Autodesk Inventor part; units mm, degrees
ref_plane "YZ Plane" through (0, 0, 0) normal (1, 0, 0) x (0, 1, 0)
ref_plane "XZ Plane" through (0, 0, 0) normal (0, 1, 0) x (-1, 0, 0)
ref_plane "XY Plane" through (0, 0, 0) normal (0, 0, 1) x (1, 0, 0)
sketch "Sketch1" plane through (0, 0, 0) normal (0, 1, 0) x (-1, 0, 0)
  line L0 (0, -27.8975) -> (20, -27.8975)
  line L1 (20, -27.8975) -> (20, -53.2975)
  line L2 (20, -53.2975) -> (0, -53.2975)
  line L3 (0, -53.2975) -> (0, -27.8975)
  point P0 (0, 0)
  dimension "d0" = 20
  dimension "d1" = 25.4
extrude "Extrusion1" add sketch "Sketch1" along normal blind 2.54
sketch "Sketch2" plane through (0, 0, -27.8975) normal (1, 0, 0) x (0, 0, -1)
  line L0 (0, 0) -> (25.4, 0)
  line L1 (0, 2.54) -> (25.4, 2.54)
  line L2 (25.4, 2.54) -> (25.4, 0)
  line L3 (25.4, 0) -> (0, 0)
  line L4 (0, 0) -> (0, 2.54)
  point P0 (-27.8975, 0)
extrude "Extrusion2" add sketch "Sketch2" along normal blind 5.08
sketch "Sketch4" plane through (-20, 0, -27.8975) normal (0, 0, 1) x (1, 0, 0)
  line L0 (25.08, 2.54) -> (25.08, 0) construction
  line L1 (25.08, 2.54) -> (20, 2.54) construction
  line L2 (0, 0) -> (25.08, 0)
  line L3 (25.08, 0) -> (20, 0)
  line L4 (0, 2.54) -> (25.08, 2.54)
  line L5 (25.08, 2.54) -> (25.08, 10.16)
  line L6 (25.08, 0) -> (25.08, -7.62)
  line L7 (20, 2.54) -> (25.08, 10.16)
  line L8 (20, 0) -> (25.08, -7.62)
  line L9 (25.08, 10.16) -> (40.32, 10.16)
  line L10 (40.32, 10.16) -> (40.32, 7.628)
  line L11 (25.08, 8.898) -> (25.08, 10.16)
  line L12 (25.08, -7.62) -> (40.32, -7.62)
  line L13 (40.32, -7.62) -> (40.32, -7.6153)
  line L14 (25.08, -7.6153) -> (25.08, -7.62)
  line L15 (40.32, 10.16) -> (42.8586, 10.16)
  line L16 (42.8586, 10.16) -> (42.8586, -7.62)
  line L17 (42.8586, -7.62) -> (40.32, -7.62)
  line L18 (40.32, -7.62) -> (40.32, 10.16)
  line L19 (40.32, -7.6177) -> (25.08, -7.6177)
  line L20 (40.32, -7.6177) -> (25.08, -7.6177)
  line L21 (25.08, -7.6177) -> (25.08, -6.3417)
  line L22 (25.08, -6.3417) -> (40.32, -6.3417)
  line L23 (40.32, -6.3417) -> (40.32, -7.6177)
  line L24 (40.32, 10.16) -> (25.08, 10.16)
  line L25 (25.08, 10.16) -> (25.08, 8.898)
  line L26 (25.08, 8.898) -> (40.32, 8.898)
  line L27 (40.32, 8.898) -> (40.32, 10.16)
  line L28 (32.7, 8.898) -> (30.1596, 8.898)
  line L29 (30.1596, 8.898) -> (30.1596, -6.3417)
  line L30 (30.1596, -6.3417) -> (32.7, -6.3417)
  line L31 (32.7, -6.3417) -> (32.7, 8.898)
  dimension "d6" = 7.62
  dimension "d7" = 2.54
  dimension "d9" = 7.62
  dimension "d10" = 15.24
  dimension "d16" = 15.24
  dimension "d30" = 17.78
extrude "Extrusion3" add sketch "Sketch4" against normal blind 25.4 contours L2 L6 L8 | L6 L22 L18 L13 L19 | L13 L18 L10 L15 L16 L17 | L29 L26 L31 L22 | L26 L5 L9 L10 | L5 L4 L7
sketch "Sketch6" plane through (22.8586, -7.62, -27.8975) normal (1, 0, 0) x (0, 0, -1)
  line L0 (25.4, 10.16) -> (25.4, 17.78)
  line L1 (0, 7.62) -> (0, 0)
  line L2 (25.4, 17.78) -> (0, 17.78)
  line L3 (0, 17.78) -> (0, 0)
  line L4 (0, 0) -> (25.4, 0)
  line L5 (25.4, 0) -> (25.4, 17.78)
  line L6 (0, 17.78) -> (0, 10.16)
  line L7 (25.4, 0) -> (0, 17.78)
  line L8 (0, 0) -> (25.4, 17.78)
  circle A0 centre (12.7, 8.89) radius 1.905
  point P0 (-27.8975, 7.62)
  dimension "d17" = 3.81
extrude "Extrusion5" cut sketch "Sketch6" against normal blind 14.2875 contours A0 L7 L8 | L8 L7 A0 | A0 L8 L7 | L7 L8 A0
sketch "Sketch8" plane through (-20, 0, -27.8975) normal (0, 0, 1) x (1, 0, 0)
  line L0 (0, 0) -> (20, 0)
  line L1 (0, 2.54) -> (20, 2.54)
  line L2 (0, 0) -> (20, 0)
  line L3 (20, 0) -> (20, 2.54)
  line L4 (20, 2.54) -> (0, 2.54)
  line L5 (0, 2.54) -> (0, 0)
extrude "Extrusion7" add sketch "Sketch8" along normal blind 50.8
sketch "Sketch10" plane through (0, 2.54, 0) normal (0, 1, 0) x (1, 0, 0)
  circle A0 centre (-10.4728, -4.8164) radius 9.779
  circle A1 centre (-10.4728, -14.5954) radius 1.905
  circle A2 centre (-10.4728, 4.9626) radius 1.905
  point P0 (0, 0)
  dimension "d31" = 19.558
  dimension "d32" = 3.81
  dimension "d33" = 3.81
extrude "Extrusion9" cut sketch "Sketch10" against normal blind 50.8 contours A2 A0 | A0 A2 | A1 A0 | A0 A1
properties part number "VbearingBracket"
Could you check a few things on this model? Use its own coordinates, in mm. A direction names the side the tool comes from. Give positions to 0.01 mm unless a question says otherwise; leave off trailing zeros. Order: outer loops, then holes, each group sorted by start corner. A loop starts at its lowest first (then second) coordinate and runs counter-clockwise, first axis right, second up. Notation, with made-up numbers: (-38.5, 52.5) -> (-3.5, 52.5) arc R13 cw to (-3.5, 72.5) -> close; hole circle Ø7 at (6, 5). An arc over 180 degrees is marked (long way). Answer in a Markdown table with one row per item. Add a question column.
Item 1: I'm going to push flat-ended pins straight in: P1, Ø16, axis at x = -9, z = 5.5, coming from the +Y side; P2, Ø3, axis at x = 1, z = -29, coming from the +Y side; P3, Ø3.5, axis at x = -10.47, z = 14.6, coming from the -Y side; P4, Ø2, axis at x = 3, y = 1, coming from the +Z side. Where does each tip first touch, or does it pass through?
Item 2: Imagine slicing it at A-A (x = 16). List the corners of the cut face in (y, z) for me.
Item 3: Please list where these lines run through material, in increasing order: probe 1 along X at (y, z) = (-3, -37.5); probe 2 along Y at (x, z) = (19.5, -29); probe 3 along Y at (x, z) = (-3.5, -36.5).
Item 4: Imagine slicing it at B-B (y = -4.5). List the corners of the cut face in (x, z) for me, and give its area (3 significant figures).
Item 5: We'd pull the mould along Y, two halves only. Please class faces 4 (the flat face through (0, 1, -3)), 5 (the flat face through (8, -6.342, -40)), 6 (the flat face through (2.504, 6.297, -40.42)): pulls with the +Y half, pulls with the -Y half, needs draft (parallel to the pull), parting line crosses it, or undercut.
Item 6: Imagine slicing it at D-D (z = 2). List the corners of the cut face in (x, y) for me.
Item 7: For faces 1 (the flat face through (8, 8.898, -40)), 2 (the flat face through (13, -7.618, -40)), 3 (the cylindrical face through (11.448, 1.842, -42.415)), which set-ups out of +Z, -Z, +X, -X, +Y, -Y let a thin tool reach every point of the face, with its end or its side?
Item 8: Imagine slicing it at C-C (y = 1.27). List the corners of the cut face in (x, z) for me (1 decimal).
Result:
| question | item | result |
|---|---|---|
| 1 | P1 | y = 2.54 |
| 1 | P2 | y = 6.29 |
| 1 | P3 | through |
| 1 | P4 | z = -27.9 |
| 2 | outline | (-7.62, -53.3) -> (-6.34, -53.3) -> (-6.34, -27.9) -> (-7.62, -27.9) -> close; (8.9, -53.3) -> (10.16, -53.3) -> (10.16, -27.9) -> (8.9, -27.9) -> close |
| 3 | probe 1 | 2 to 5.08, 10.16 to 12.7, 20.32 to 22.86 |
| 3 | probe 2 | -7.62 to -6.34, 8.9 to 10.16 |
| 3 | probe 3 | 0 to 2.54 |
| 4 | outline | (3, -53.3) -> (5.08, -53.3) -> (5.08, -27.9) -> (3, -27.9) -> close; (10.16, -53.3) -> (12.7, -53.3) -> (12.7, -27.9) -> (10.16, -27.9) -> close; (20.32, -53.3) -> (22.86, -53.3) -> (22.86, -27.9) -> (20.32, -27.9) -> close |
| 4 | area | 182 mm2 |
| 5 | face 4 | needs draft |
| 5 | face 5 | undercut |
| 5 | face 6 | pulls with the +Y half |
| 6 | outline | (-20, 0) -> (0, 0) -> (0, 2.54) -> (-20, 2.54) -> close |
| 7 | face 1 | +Z, -Z |
| 7 | face 2 | +Z, -Z, +X, -X, -Y |
| 7 | face 3 | +X |
| 8 | outline | (-20, -53.3) -> (5.1, -53.3) -> (5.1, -27.9) -> (0, -27.9) -> (0, 22.9) -> (-20, 22.9) -> close; (10.2, -53.3) -> (12.7, -53.3) -> (12.7, -42.5) -> (10.2, -42.5) -> close; (10.2, -38.7) -> (12.7, -38.7) -> (12.7, -27.9) -> (10.2, -27.9) -> close; (20.3, -53.3) -> (22.9, -53.3) -> (22.9, -42.5) -> (20.3, -42.5) -> close; (20.3, -38.7) -> (22.9, -38.7) -> (22.9, -27.9) -> (20.3, -27.9) -> close; hole circle Ø3.8 at (-10.5, -5); hole circle Ø3.8 at (-10.5, 14.6) |
